from build123d import *

# Parameters (mm, degrees)
F0_W           = 25.4
F0_H           = 25.4
F1_DEPTH       = 25.4
F5_D           = 5.1054
F5_DEPTH       = 16.51
F5_TIP         = 1.5338169022
F5_ON_F3_D     = 5.1054
F5_ON_F3_DEPTH = 16.51
F5_ON_F3_TIP   = 1.5338169022
F5_ON_F4_D     = 5.1054
F5_ON_F4_DEPTH = 16.51
F5_ON_F4_TIP   = 1.5338169022


with BuildPart() as f1:
    # F0 (on Top) → F1 (new body)
    with BuildSketch(Plane.XY):
        Rectangle(F0_W, F0_H)
    extrude(amount=F1_DEPTH)

    # F5
    with Locations(Plane.XY.offset(25.4)):
        with Locations((0, 0)):
            Hole(F5_D / 2, depth=F5_DEPTH)
            with Locations((0, 0, -(F5_DEPTH + F5_TIP / 2))):  # 118° drill point
                Cone(0, F5_D / 2, F5_TIP, mode=Mode.SUBTRACT)

    # F5 on F3
    with Locations(Plane.YZ.offset(12.7)):
        with Locations((0, 12.7)):
            Hole(F5_ON_F3_D / 2, depth=F5_ON_F3_DEPTH)
            with Locations((0, 0, -(F5_ON_F3_DEPTH + F5_ON_F3_TIP / 2))):  # 118° drill point
                Cone(0, F5_ON_F3_D / 2, F5_ON_F3_TIP, mode=Mode.SUBTRACT)

    # F5 on F4
    with Locations(Plane(origin=(0, 12.7, 0), x_dir=(-1, 0, 0), z_dir=(0, 1, 0))):
        with Locations((0, 12.7)):
            Hole(F5_ON_F4_D / 2, depth=F5_ON_F4_DEPTH)
            with Locations((0, 0, -(F5_ON_F4_DEPTH + F5_ON_F4_TIP / 2))):  # 118° drill point
                Cone(0, F5_ON_F4_D / 2, F5_ON_F4_TIP, mode=Mode.SUBTRACT)


solid = f1.part
Could you check a few things on this model? Use its own coordinates, in mm. A direction names the side the tool comes from. Coordinates: 2 decimals unless noted, no trailing zeros. Order: outer loops, then holes, each group sorted by start corner. A loop starts at its lowest first (then second) coordinate and runs counter-clockwise, first axis right, second up.
Q1. Suppose I cut it at A-A on y = 7. Please give me the cut outline in (x, z), and give its area (3 significant figures).
Q2. Will these pins go through, and if not, where does the flat tip stop? pin 1 (4 mm diameter, centred on x = 0, y = 0, fed in from -Z); pin 2 (4.5 mm diameter, centred on x = 0, z = 12.7, fed in from +Y); pin 3 (4.5 mm diameter, centred on y = 0, z = 12.7, fed in from +X).
Q3. Thinking about a two-plate mould opening in Z: for faces 5 (the cylindrical face through (-3.044, 1.881, 14.425)), 6 (the flat face through (12.7, 3, 13)), 7 (the conical face through (0.41, -0.17, 7.623)), which applies, released by +Z, released by -Z, zero draft, split by the parting line, or undercut?
Q4. Which directions (+Z, -Z, +X, -X, +Y, -Y) give clear straight access to the entire face, cutting with the end or side of a thin tool? Please do faces 1 (the cylindrical face through (-1.881, -3.044, 14.425)), 2 (the flat face through (3, 0, 25.4)), 3 (the cylindrical face through (2.55, 0.11, 19.88)), 4 (the cylindrical face through (7.18, 2.55, 12.81)).
Q5. Please list where these lines run through material, in increasing order: L1, parallel to Z at x = 5.75, y = 0; L2, parallel to X at y = -3.2, z = 12.7.
Answer:
1. outline: (-12.7, 0) - (12.7, 0) - (12.7, 25.4) - (-12.7, 25.4) - close; hole circle Ø5.11 at (0, 12.7)
1. area: 625 mm2
2. pin 1: stops at z = 0
2. pin 2: stops at y = -3.99
2. pin 3: stops at x = -3.99
3. face 5: undercut
3. face 6: zero draft
3. face 7: released by +Z
4. face 1: +Y
4. face 2: +Z, +X, -X, +Y, -Y
4. face 3: +Z
4. face 4: +X
5. L1: z = 0 to 10.15, 15.25 to 25.4
5. L2: x = -12.7 to -2.55, 2.55 to 12.7
